Check sheet for the modelled part. Datum: model origin and axes. Units: mm. Face numbers are marked on the shaded views. A direction names the side the tool comes from. Round coordinates to 2 decimals unless told otherwise and drop trailing zeros. Write each loop counter-clockwise with the first axis right and the second up, starting at its lowest first coordinate (ties: lowest second). Pieces come first, ordered by that corner, then holes.
Item 1: Cross-section at B-B on x = 34.85. Enter the section's corners in (y, z).
Item 2: Cross-section at A-A on y = 41.5. Enter the section's corners in (x, z), plus the area to 3 significant figures.
Item 3: Material ranges on line 1 (Z direction, x = 14.85, y = 44.1); line 2 (X direction, y = 44.5, z = -36); line 3 (X direction, y = 23, z = -25), recorded low to high.
Item 4: Cross-section at C-C on z = -14.88. Enter the section's corners in (x, y), plus the area to 3 significant figures.
Item 5: Go/stop test with flat-tipped pins: pin 1 Ø3.5 at (y, z) = (16.97, -36.97) entering from +X; pin 2 Ø2 at (x, z) = (27.5, -37) entering from -Y. Record where each tip stops, or that it passes through.
Item 6: Tool access check on the marked faces 1 and 2. Record the directions out of +Z, -Z, +X, -X, +Y, -Y that give a thin tool (end or side, any length) a straight path to the whole face; none if there is none.
Item 7: Release check for a two-part mould opening along X. For the marked faces 3, 4, 5 and 6 record: +X half, -X half, draft (parallel to the pull), parting line (faces both ways), or undercut.
Item 8: Cross-section at D-D on y = 32.97. Enter the section's corners in (x, z), plus the area to 3 significant figures.
Autodesk Inventor part; units mm, degrees
ref_plane "Arbeitsebene2" through (41.82, 8, -41.82) normal (0, 0, 1) x (1, 0, 0)
ref_plane "YZ Plane" through (0, 0, 0) normal (1, 0, 0) x (0, 1, 0)
ref_plane "XZ Plane" through (0, 0, 0) normal (0, 1, 0) x (-1, 0, 0)
ref_plane "Arbeitsebene1" through (49.7, 8, -8.38) normal (0, 0, -1) x (-1, 0, 0)
sketch "Skizze1" plane through (49.7, 8, -8.38) normal (0, 0, -1) x (-1, 0, 0)
  line L0 (2, 0) -> (2, 41.6)
  line L1 (7.88, 0) -> (2, 0)
  line L2 (7.88, 34.1) -> (7.88, 0)
  line L3 (47.7, 34.1) -> (7.88, 34.1)
  line L4 (47.7, 41.6) -> (47.7, 34.1)
  line L5 (2, 41.6) -> (47.7, 41.6)
  line L6 (40.85, 0) -> (40.85, -4.62)
  line L7 (40.85, -4.62) -> (8.85, -4.62)
  line L8 (8.85, -4.62) -> (8.85, 0)
  line L9 (2, 0) -> (8.85, 0)
  line L10 (2, -7.5) -> (2, 0)
  line L11 (47.7, -7.5) -> (2, -7.5)
  line L12 (47.7, 34.1) -> (47.7, -7.5)
  line L13 (41.82, 34.1) -> (47.7, 34.1)
  line L14 (41.82, 0) -> (41.82, 34.1)
  line L15 (40.85, 0) -> (41.82, 0)
  line L16 (10.35, -3.12) -> (10.35, 34.38)
  line L17 (39.35, 34.38) -> (39.35, -3.12)
  line L18 (39.35, 34.38) -> (39.35, -3.12)
  line L19 (39.35, 34.38) -> (10.35, 34.38)
  line L20 (10.35, -3.12) -> (10.35, 34.38)
  line L21 (39.35, -3.12) -> (10.35, -3.12)
  line L22 (10.35, -3.12) -> (39.35, -3.12) construction
  line L23 (39.35, -3.12) -> (39.35, 34.38) construction
  line L24 (39.35, 34.38) -> (10.35, 34.38) construction
  line L25 (10.35, 34.38) -> (10.35, -3.12) construction
  line L26 (10.05, 34.68) -> (39.65, 34.68) construction
  line L27 (39.65, 34.68) -> (39.65, -3.42) construction
  line L28 (39.65, -3.42) -> (10.05, -3.42) construction
  line L29 (10.05, -3.42) -> (10.05, 34.68) construction
  line L30 (10.05, 0.3432) -> (7.98, 0.3432)
  line L31 (7.98, 0.3432) -> (7.98, 37.6)
  line L32 (7.98, 37.6) -> (10.05, 37.6)
  line L33 (10.05, 37.6) -> (10.05, 0.3432)
  line L34 (10.05, 37.6) -> (24.85, 37.6)
  line L35 (24.85, 37.6) -> (24.85, 34.68)
  line L36 (24.85, 34.68) -> (10.05, 34.68)
  line L37 (10.05, 34.68) -> (10.05, 37.6)
  point P0 (49.7, -8)
  point P1 (24.85, 34.68)
  dimension "d1" = 0.3
  dimension "d2" = 0.1
  dimension "d3" = 4
ref_plane "Arbeitsebene2" through (41.82, 8, -41.82) normal (0, 0, 1) x (1, 0, 0)
extrude "Extrusion1" add sketch "Skizze1" along normal blind 33 contours L31 L32 L33 L3 | L3 L33 L30 L31 | L33 L34 L35 L36
sketch "Skizze2" plane through (41.72, 8.3432, -8.38) normal (1, 0, 0) x (0, 0, -1)
  circle A0 centre (12.6606, 8.6268) radius 1.4
  circle A1 centre (28.5855, 24.6268) radius 1.4
  circle A2 centre (28.5855, 8.6268) radius 1.4
  point P0 (-8.38, -8.3432)
extrude "Extrusion2" cut sketch "Skizze2" against normal blind 33
sketch "Skizze3" plane through (24.85, 45.6, -8.38) normal (0, 1, 0) x (1, 0, 0)
  line L0 (0, 0) -> (16.87, 0)
  line L1 (16.87, 0) -> (16.87, 33)
  line L2 (0, 33) -> (16.87, 33)
  line L3 (0, 0) -> (0, 33)
  line L4 (-10, 6.5) -> (10, 6.5)
  line L5 (10, 6.5) -> (10, 26.5)
  line L6 (10, 26.5) -> (-10, 26.5)
  line L7 (-10, 26.5) -> (-10, 6.5)
  line L8 (-10, 6.5) -> (10, 26.5) construction
  line L9 (10, 6.5) -> (-10, 26.5) construction
  circle A0 centre (10, 26.5) radius 1.4
  circle A1 centre (10, 6.5) radius 1.4
  point P0 (-24.85, -8.38)
  point P1 (0, 16.5)
  dimension "d8" = 20
  dimension "d9" = 20
  dimension "d10" = 2.8
  dimension "d11" = 2.8
extrude "Extrusion3" cut sketch "Skizze3" against normal blind 33 contours A1 L5 L4 | L4 L5 A1 | A0 L5 L6 | L6 L5 A0
mirror "Spiegeln1" about plane through (24.85, 42.68, -8.38) normal (-1, 0, 0) of "Extrusion1", "Extrusion2", "Extrusion3"
properties part number "Assembly_Cube_Laser_Multicolour_insert_v3"
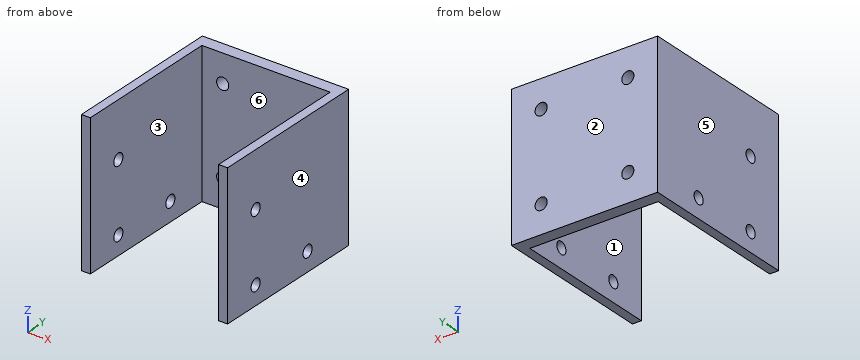
Response values:
1. outline: (42.68, -41.38) - (45.6, -41.38) - (45.6, -36.28) - (42.68, -36.28) - close; (42.68, -33.48) - (45.6, -33.48) - (45.6, -16.28) - (42.68, -16.28) - close; (42.68, -13.48) - (45.6, -13.48) - (45.6, -8.38) - (42.68, -8.38) - close
2. outline: (7.98, -41.38) - (10.05, -41.38) - (10.05, -8.38) - (7.98, -8.38) - close; (39.65, -41.38) - (41.72, -41.38) - (41.72, -8.38) - (39.65, -8.38) - close
2. area: 137 mm2
3. line 1: z = -41.38 to -36.28, -33.48 to -16.28, -13.48 to -8.38
3. line 2: x = 7.98 to 14.01, 15.69 to 34.01, 35.69 to 41.72
3. line 3: x = 7.98 to 10.05, 39.65 to 41.72
4. outline: (7.98, 8.34) - (10.05, 8.34) - (10.05, 42.68) - (13.45, 42.68) - (13.45, 45.6) - (7.98, 45.6) - close; (16.25, 42.68) - (33.45, 42.68) - (33.45, 45.6) - (16.25, 45.6) - close; (36.25, 42.68) - (39.65, 42.68) - (39.65, 8.34) - (41.72, 8.34) - (41.72, 45.6) - (36.25, 45.6) - close
4. area: 224 mm2
5. pin 1: stops at x = 41.72
5. pin 2: stops at y = 42.68
6. face 1: +Z, -Z, -Y
6. face 2: +Z, -Z, +X, -X, +Y
7. face 3: undercut
7. face 4: +X half
7. face 5: -X half
7. face 6: undercut
8. outline: (7.98, -41.38) - (10.05, -41.38) - (10.05, -38.37) - (7.98, -38.37) - close; (7.98, -35.57) - (10.05, -35.57) - (10.05, -8.38) - (7.98, -8.38) - close; (39.65, -41.38) - (41.72, -41.38) - (41.72, -38.37) - (39.65, -38.37) - close; (39.65, -35.57) - (41.72, -35.57) - (41.72, -8.38) - (39.65, -8.38) - close
8. area: 125 mm2
